Work out the finished part from the listing and answer in its coordinate system (mm). Coordinates: 2 decimals unless noted, no trailing zeros. Write each loop counter-clockwise with the first axis right and the second up, starting at its lowest first coordinate (ties: lowest second). Pieces come first, ordered by that corner, then holes. Notation, with made-up numbers: (56.25, 67.25) - (88.25, 67.25) arc R12 ccw to (88.25, 87.25) - close; hole circle Ø9 at (41.25, 4.5). An arc over 180 degrees is marked (long way). Use a Markdown table: item, result. Add a question column.
(1) The part is cut by section A-A, the plane y = 1.8. State how many separate pieces and enclosed holes the cut face has, then the cut area to 3 significant figures.
(2) The part is cut by section C-C, the plane x = 31.75. Give the vertices of the cut face in (y, z).
(3) The part is cut by section D-D, the plane z = 60. Give the vertices of the cut face in (x, y), then the cut area to 3 significant figures.
(4) Find the intervals of material crossed by line 1 (X direction, y = 3.3, z = -63.5); line 2 (X direction, y = 2.8, z = 19.5) (3 decimals); line 3 (Z direction, x = -31.75, y = 1.3), in increasing order. Write a range as from..to.
(5) Given pin 1 Ø1 at (x, y) = (-23, 1.5) entering from -Z; pin 2 Ø3 at (y, z) = (2, 50.5) entering from -X; pin 3 Ø1 at (y, z) = (3.5, 54.5) entering from +X, each flat-ended and moving along its own axis, determine where each tip first touches the part or whether it passes through.
(6) The part is cut by section B-B, the plane z = -63.5. Give the vertices of the cut face in (x, y).
(7) For a pull along Z with two mould halves and no side action, classify faces 1 (the face through (-19.946, 2.535, 19.426)), 2 (the face through (39.99, 2.46, -65.78)), 3 (the face through (1, 0, 1)) as released by +Z, released by -Z, zero draft, split by the parting line, or undercut.
Autodesk Inventor part; units mm, degrees
ref_plane "YZ Plane" through (0, 0, 0) normal (1, 0, 0) x (0, 1, 0)
ref_plane "XZ Plane" through (0, 0, 0) normal (0, 1, 0) x (-1, 0, 0)
ref_plane "XY Plane" through (0, 0, 0) normal (0, 0, 1) x (1, 0, 0)
sketch "Sketch1" plane through (0, 0, 0) normal (0, 1, 0) x (-1, 0, 0)
  line L0 (-22.225, 73.025) -> (22.225, 73.025)
  line L1 (47.625, 47.625) -> (47.625, -47.625)
  line L2 (22.225, -73.025) -> (-22.225, -73.025)
  line L3 (-47.625, -47.625) -> (-47.625, 47.625)
  line L4 (-47.625, 73.025) -> (47.625, -73.025) construction
  line L5 (47.625, 73.025) -> (-47.625, -73.025) construction
  arc A0 (22.225, -73.025) -> (47.625, -47.625) centre (22.225, -47.625) ccw
  arc A1 (-47.625, -47.625) -> (-22.225, -73.025) centre (-22.225, -47.625) ccw
  arc A2 (-22.225, 73.025) -> (-47.625, 47.625) centre (-22.225, 47.625) ccw
  arc A3 (47.625, 47.625) -> (22.225, 73.025) centre (22.225, 47.625) ccw
  point P0 (0, 0)
  dimension "d11" = 95.25
  dimension "d12" = 146.05
  dimension "d13" = 25.4
extrude "Extrusion1" add sketch "Sketch1" along normal blind 5
sketch "Sketch3" plane through (0, 5, 0) normal (0, 1, 0) x (1, 0, 0)
  circle A0 centre (-31.75, -63.5) radius 1.7
  line L0 (-47.625, 47.625) -> (-47.625, -47.625) construction
  line L1 (-47.625, 0) -> (47.625, 0) construction
  line L2 (47.625, -47.625) -> (47.625, 47.625) construction
  line L3 (0, -72.5867) -> (0, 73.025) construction
  line L4 (22.225, 73.025) -> (-22.225, 73.025) construction
  circle A1 centre (-31.75, 63.5) radius 1.7
  circle A2 centre (31.75, -63.5) radius 1.7
  circle A3 centre (31.75, 63.5) radius 1.7
  point P0 (0, 0)
  dimension "d14" = 3.4
  dimension "d15" = 63.5
  dimension "d16" = 31.75
extrude "Standoffs" cut sketch "Sketch3" against normal through all
sketch "Sketch4" plane through (0, 5, 0) normal (0, 1, 0) x (1, 0, 0)
  circle A0 centre (-20.8597, -20.8597) radius 1.7
  line L0 (-47.625, 47.625) -> (-47.625, -47.625) construction
  line L1 (-47.625, 0) -> (47.625, 0) construction
  line L2 (47.625, -47.625) -> (47.625, 47.625) construction
  line L3 (-22.225, -73.025) -> (22.225, -73.025) construction
  line L4 (0, -73.025) -> (0, 73.025) construction
  line L5 (22.225, 73.025) -> (-22.225, 73.025) construction
  line L6 (-20.8597, -20.8597) -> (0, 0) construction
  circle A1 centre (-20.8597, 20.8597) radius 1.7
  circle A2 centre (20.8597, -20.8597) radius 1.7
  circle A3 centre (20.8597, 20.8597) radius 1.7
  dimension "d19" = 3.4
  dimension "d20" = 45
  dimension "d21" = 29.5
extrude "LiDAR Mounts" cut sketch "Sketch4" against normal through all
equation "\"d3\" = hardboard_thickness"
equation "\"d14\" = m3_clearance"
equation "\"d19\" = m3_clearance"
equation "\"m3_heat_set_insert\" = 4"
equation "\"m3_clearance\" = 3.4"
equation "\"m3_heat_set_depth\" = 7"
equation "\"robot_diameter\" = 354"
equation "\"hardboard_thickness\" = 5"
properties part number "LiDAR_plate"
Model answer:
| question | item | result |
|---|---|---|
| 1 | separate pieces | 1 |
| 1 | enclosed holes | 8 |
| 1 | area | 13,300 mm^2 |
| 2 | outline | (0, -71.17) - (5, -71.17) - (5, -65.2) - (0, -65.2) - close; (0, -61.8) - (5, -61.8) - (5, 61.8) - (0, 61.8) - close; (0, 65.2) - (5, 65.2) - (5, 71.17) - (0, 71.17) - close |
| 3 | outline | (-44.41, 0) - (44.41, 0) - (44.41, 5) - (-44.41, 5) - close |
| 3 | area | 444 mm^2 |
| 4 | line 1 | -42.05..-33.45, -30.05..30.05, 33.45..42.05 |
| 4 | line 2 | -47.625..-21.88, -19.839..19.839, 21.88..47.625 |
| 4 | line 3 | -71.17..-65.2, -61.8..61.8, 65.2..71.17 |
| 5 | pin 1 | z = -73.02 |
| 5 | pin 2 | x = -47.59 |
| 5 | pin 3 | x = 46.81 |
| 6 | outline | (-42.05, 0) - (-33.45, 0) - (-33.45, 5) - (-42.05, 5) - close; (-30.05, 0) - (30.05, 0) - (30.05, 5) - (-30.05, 5) - close; (33.45, 0) - (42.05, 0) - (42.05, 5) - (33.45, 5) - close |
| 7 | face 1 | undercut |
| 7 | face 2 | released by -Z |
| 7 | face 3 | zero draft |
